from build123d import *

# Parameters (mm, degrees)
F2_T     = -6
F4_W     = 30
F4_H     = 50
F6_R     = 3
F7_DEPTH = 2


# Not quite as in the source:
# - a pattern or mirror of a feature is missing from the dataset's text; its kind, count and spacing are read off the source's solid


with BuildPart() as f1:
    # F0 (on Front) → F1 (revolve)
    with BuildSketch(Plane.XZ):
        with BuildLine():
            Line((0, 0), (-100, 0))
            ThreePointArc((-100, 0), (-96.5925826289, -25.8819045103), (-86.6025403784, -50))
            Line((-86.6025403784, -50), (0, -50))
            Line((0, -50), (0, 0))
        make_face()
    revolve(axis=Axis((0, 0, -25), (0, 0, -1)))

    # F2
    f2_openings = [f1.faces().sort_by_distance(p)[0] for p in [
        (0, 0, 0),
        (0, 0, -50),
    ]]
    offset(amount=F2_T, openings=f2_openings)

    # F4 (on offset) → F5 (join, up to the next surface of F1)
    with BuildSketch(Plane.XZ.offset(-58)):
        with Locations((0, -25)):
            Rectangle(F4_W, F4_H)
    f5 = extrude(until=Until.NEXT, dir=(0, 1, 0))

    # F5_copies: F5 across plane
    add(f5.mirror(Plane(origin=(0, 0, 0), x_dir=(0, 0, -1), z_dir=(0, -1, 0))))

    # F6 (on face) → F7 (cut)
    with BuildSketch(Plane.XZ.offset(-58)):
        with Locations((0, -25)):
            Circle(F6_R)
    f7 = extrude(amount=-F7_DEPTH, mode=Mode.SUBTRACT)

    # F7_copies: F7 across plane
    add(f7.mirror(Plane(origin=(0, 0, 0), x_dir=(0, 0, -1), z_dir=(0, -1, 0))), mode=Mode.SUBTRACT)


solid = f1.part
Check sheet for the modelled part. Datum: model origin and axes. Units: mm. A direction names the side the tool comes from. Round coordinates to 2 decimals unless told otherwise and drop trailing zeros. Order: outer loops, then holes, each group sorted by start corner. A loop starts at its lowest first (then second) coordinate and runs counter-clockwise, first axis right, second up.
(1) Draft check along X on faces 1 (the flat face through (15, 75, -25)), 2 (the flat face through (0, 60, 0)). Enter one of: pulls with the +X half, pulls with the -X half, needs draft (parallel to the pull), parting line crosses it, or undercut.
(2) Cross-section at B-B, the plane y = -67. Enter the section's corners in (x, z), and give its area (3 significant figures).
(3) Access from +Z, -Z, +X, -X, +Y, -Y to the whole of each face (thin tool, end or side, straight path). Record for faces 3 (the flat face through (-15, 75, -25)), 4 (the flat face through (0, 65, -50)), 5 (the flat face through (-4, 58, -25)), 6 (the flat face through (0, -60, -25)).
(4) Cross-section at A-A, the plane x = 0. Enter the section's corners in (y, z), and give its area (3 significant figures).
(5) Scan lines: probe 1 along Z at (x, y) = (0, 58.4); probe 2 along X at (y, z) = (-71, -11.5); probe 3 along X at (y, z) = (-73, -16). Record each from-to range of solid material in increasing order.
(6) Cross-section at C-C, the plane z = -25. Enter the section's corners in (x, y), and give its area (3 significant figures).
(7) Cross-section at D-D, the plane y = 13. Enter the section's corners in (x, z).
(8) Go/stop test with flat-tipped pins: P1, Ø5, axis at y = 78, z = -22, coming from the -X side; P2, Ø8, axis at y = -79.5, z = -42.5, coming from the -X side; P3, Ø10, axis at y = -48, z = -19, coming from the +X side. Record where each tip stops, or that it passes through.
Check sheet entries:
1. face 1: undercut
1. face 2: needs draft
2. outline: (-74.24, 0) arc R74.24 ccw to (-54.87, -50) - (-42.98, -50) arc R65.93 cw to (-65.93, 0) - close; (-15, -50) - (15, -50) - (15, 0) - (-15, 0) - close; (42.98, -50) - (54.87, -50) arc R74.24 ccw to (74.24, 0) - (65.93, 0) arc R65.93 cw to start
2. area: 2,430 mm2
3. face 3: +Z
3. face 4: -Z, +X, -X, +Y, -Y
3. face 5: +Z, -Z
3. face 6: none
4. outline: (-100, 0) arc R100 ccw to (-86.6, -50) - (-58, -50) - (-58, -28) - (-60, -28) - (-60, -22) - (-58, -22) - (-58, 0) - close; (58, -50) - (86.6, -50) arc R100 ccw to (100, 0) - (58, 0) - (58, -22) - (60, -22) - (60, -28) - (58, -28) - close
4. area: 3,740 mm2
5. probe 1: z = -50 to -28, -22 to 0
5. probe 2: x = -69.47 to -60.52, -15 to 15, 60.52 to 69.47
5. probe 3: x = -66.45 to -57.02, -15 to 15, 57.02 to 66.45
6. outline: circle Ø193.65 at (0, 0); hole (-15, -89.36) - (-15, -58) - (-3, -58) - (-3, -60) - (3, -60) - (3, -58) - (15, -58) - (15, -89.36) arc R90.61 ccw to (15, 89.36) - (15, 58) - (3, 58) - (3, 60) - (-3, 60) - (-3, 58) - (-15, 58) - (-15, 89.36) arc R90.61 ccw to start
6. area: 5,560 mm2
7. outline: (-99.15, 0) arc R99.15 ccw to (-85.62, -50) - (-78.53, -50) arc R93.1 cw to (-93.1, 0) - close; (78.53, -50) - (85.62, -50) arc R99.15 ccw to (99.15, 0) - (93.1, 0) arc R93.1 cw to start
8. P1: stops at x = -61.89
8. P2: stops at x = -50.78
8. P3: stops at x = 88.47
